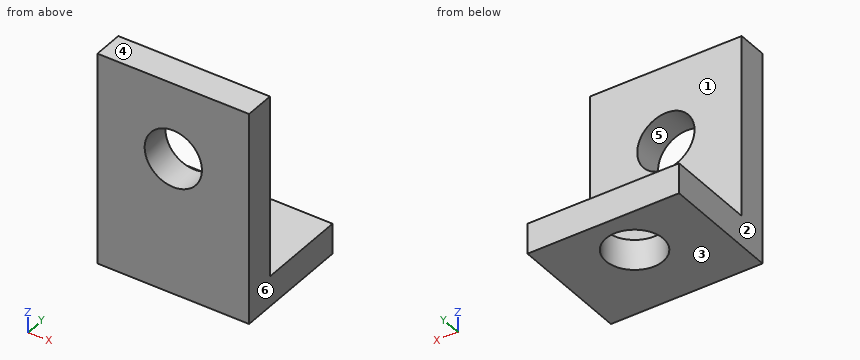
```python
from build123d import *

# Parameters (mm, degrees)
SKETCH2_W               = 10.16
SKETCH2_H               = 10.16
BOSS_EXTRUDE1_DEPTH     = 38.1
CUT_EXTRUDE1_DEPTH      = 41.719297636
CUT_EXTRUDE1_DEPTH_BACK = 38.1
SKETCH3_W               = 7.62
SKETCH3_H               = 7.62
M4_CLEARANCE_HOLE2_D    = 4.8
SKETCH13_W              = 38.1
SKETCH13_H              = 2.54
BOSS_EXTRUDE2_DEPTH     = 7.62
M4_CLEARANCE_HOLE3_D    = 4.8
CUT_EXTRUDE2_REACH      = 45.255
SKETCH17_W              = 25.4
SKETCH17_H              = 10.16


with BuildPart() as part:
    # Sketch2 → Boss-Extrude1 (new body)
    with BuildSketch(Plane(origin=(0, 0, 0), x_dir=(0, 0, -1), z_dir=(1, 0, 0))):
        with Locations((5.08, 5.08)):
            Rectangle(SKETCH2_W, SKETCH2_H)
    extrude(amount=BOSS_EXTRUDE1_DEPTH)

    # Sketch3 → Cut-Extrude1 (cut, two sides: drawn at the far end of the back side and taken through both)
    with BuildSketch(Plane(origin=(38.1, 0, 0), x_dir=(0, 0, -1), z_dir=(1, 0, 0)).offset(-CUT_EXTRUDE1_DEPTH_BACK)):
        with Locations((3.81, 6.35)):
            Rectangle(SKETCH3_W, SKETCH3_H)
    extrude(amount=CUT_EXTRUDE1_DEPTH + CUT_EXTRUDE1_DEPTH_BACK, mode=Mode.SUBTRACT)

    # M4 Clearance Hole2 (through all)
    with Locations(Plane.XY.offset(-7.62)):
        with Locations((6.35, 6.35), (31.75, 6.35)):
            Hole(M4_CLEARANCE_HOLE2_D / 2)

    # Sketch13 → Boss-Extrude2 (add)
    with BuildSketch(Plane.XY):
        with Locations((19.05, 1.27)):
            Rectangle(SKETCH13_W, SKETCH13_H)
    extrude(amount=BOSS_EXTRUDE2_DEPTH)

    # M4 Clearance Hole3 (through all)
    with Locations(Plane(origin=(0, 2.54, 0), x_dir=(1, 0, 0), z_dir=(0, 1, 0))):
        with Locations((6.35, -1.27), (31.75, -1.27)):
            Hole(M4_CLEARANCE_HOLE3_D / 2)

    # Cut-Extrude2: up to this face of the body (flat: up to its plane)
    cut_extrude2_end = Plane(part.part.faces().sort_by_distance((19.05, 1.27, 7.62))[0])
    # Sketch17 → Cut-Extrude2 (cut, up to the picked face)
    with BuildSketch(Plane(origin=(0, 0, -10.16), x_dir=(-1, 0, 0), z_dir=(0, 0, -1)), mode=Mode.PRIVATE) as cut_extrude2_sk1:
        with Locations((-25.4, 5.08)):
            Rectangle(SKETCH17_W, SKETCH17_H)
    cut_extrude2_tool1 = split(extrude(cut_extrude2_sk1.sketch, amount=-CUT_EXTRUDE2_REACH, mode=Mode.PRIVATE), bisect_by=cut_extrude2_end, keep=Keep.BOTH, mode=Mode.PRIVATE)
    add(cut_extrude2_tool1.solids().sort_by(Axis((25.4, 5.08, -10.16), (0, 0, 1)))[0], mode=Mode.SUBTRACT)


solid = part.part
```
Here's how the part is built. I have some questions about the finished solid (model axes, mm). Face numbers are marked on the shaded views. A direction names the side the tool comes from. Coordinates: 2 decimals unless noted, no trailing zeros. Order: outer loops, then holes, each group sorted by start corner. A loop starts at its lowest first (then second) coordinate and runs counter-clockwise, first axis right, second up.
Item 1: I need wall thicknesses on probe 1 along Z at (x, y) = (11.5, 4.5); probe 2 along Y at (x, z) = (9.25, -4); probe 3 along X at (y, z) = (1.75, -0.5). Which ranges of each line are inside material? Lowest first, please.
Response values:
probe 1: z = -10.16 to -7.62
probe 2: y = 0 to 2.54
probe 3: x = 0 to 4.73, 7.97 to 12.7
Item 2: Which directions (+Z, -Z, +X, -X, +Y, -Y) give clear straight access to the entire face, cutting with the end or side of a thin tool? Please do the marked faces 1 and 2.
Response values:
face 1: +Z, +X, -X, +Y
face 2: +Z, -Z, -X, +Y, -Y
Item 3: If we section it at C-C, the plane y = 6.35: List the corners of the cut face in (x, z) for me.
Response values:
outline: (0, -10.16) - (3.95, -10.16) - (3.95, -7.62) - (0, -7.62) - close; (8.75, -10.16) - (12.7, -10.16) - (12.7, -7.62) - (8.75, -7.62) - close
Item 4: If we section it at A-A, the plane z = 1.27: List the corners of the cut face in (x, y) for me.
Response values:
outline: (0, 0) - (3.95, 0) - (3.95, 2.54) - (0, 2.54) - close; (8.75, 0) - (12.7, 0) - (12.7, 2.54) - (8.75, 2.54) - close
Item 5: If we section it at D-D, the plane z = -8.5: List the corners of the cut face in (x, y) for me, then the cut area to 3 significant figures.
Response values:
outline: (0, 0) - (12.7, 0) - (12.7, 10.16) - (0, 10.16) - close; hole circle Ø4.8 at (6.35, 6.35)
area: 111 mm2
Item 6: I'm going to push flat-ended pins straight in: pin 1 Ø6 at (x, y) = (6.35, 6.35) entering from +Z; pin 2 Ø1 at (x, z) = (7, 0.5) entering from +Y; pin 3 Ø5 at (x, y) = (6.5, 5) entering from +Z; pin 4 Ø7.5 at (x, z) = (6.35, 1.27) entering from +Y. Where does each tip first touch, or does it pass through?
Response values:
pin 1: stops at z = -7.62
pin 2: passes through
pin 3: stops at z = 7.62
pin 4: stops at y = 2.54
Item 7: If we section it at B-B, the plane x = 6.35: List the corners of the cut face in (y, z) for me.
Response values:
outline: (0, -10.16) - (3.95, -10.16) - (3.95, -7.62) - (2.54, -7.62) - (2.54, -1.13) - (0, -1.13) - close; (0, 3.67) - (2.54, 3.67) - (2.54, 7.62) - (0, 7.62) - close; (8.75, -10.16) - (10.16, -10.16) - (10.16, -7.62) - (8.75, -7.62) - close
Item 8: Thinking about a two-plate mould opening in Z: for the marked faces 3, 4, 5 and 6, which applies, pulls with the +Z half, pulls with the -Z half, needs draft (parallel to the pull), parting line crosses it, or undercut?
Response values:
face 3: pulls with the -Z half
face 4: pulls with the +Z half
face 5: undercut
face 6: needs draft
